Part print with two shaded views. Sizes in mm from the minimum x, y, z corner. A direction names the side the tool comes from. Coordinates: 2 decimals unless noted, no trailing zeros. Loops run counter-clockwise (first coordinate to the right, second up) from the corner with the lowest first, then second, coordinate; pieces in that order, holes last. Notation, with made-up numbers: (9.25, 19) -> (60.25, 19) arc R21 ccw to (60.25, 29) -> close; hole circle Ø5 at (-35, 54.5). An arc over 180 degrees is marked (long way). Answer as a JSON object with one key per item and string values. Group by question number.
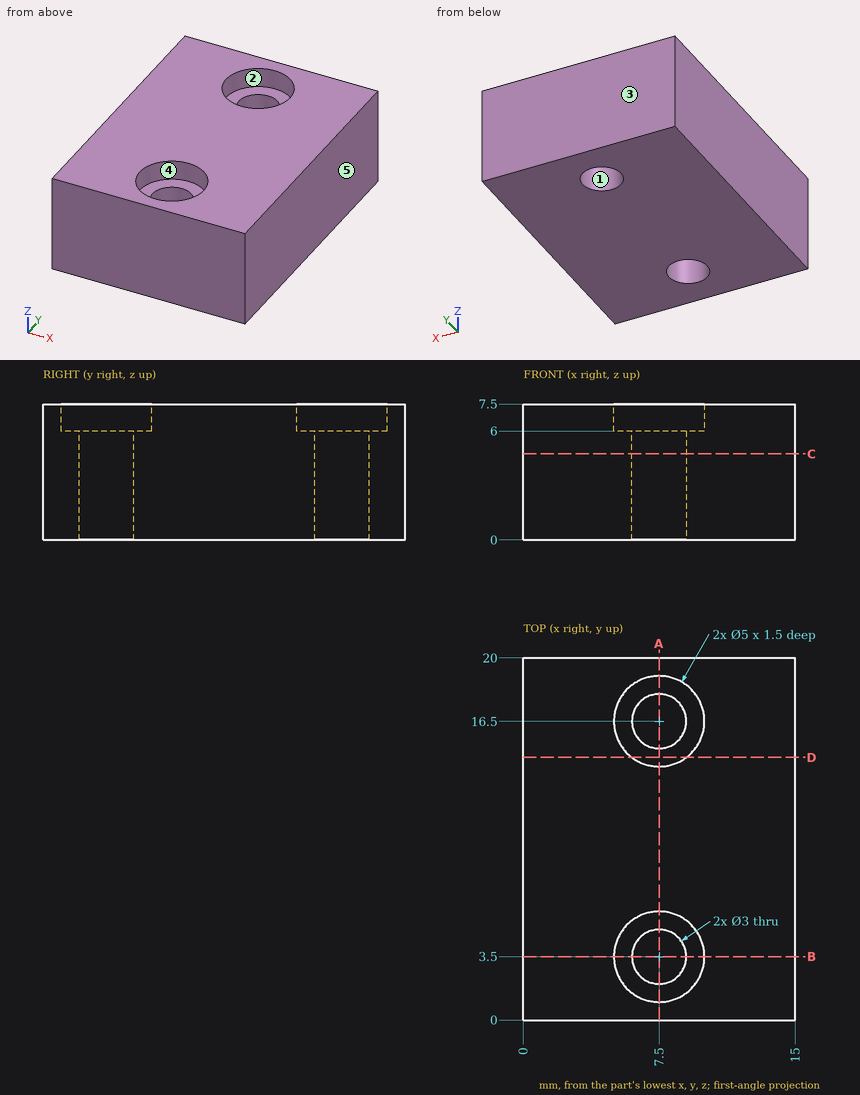
Item 1: Band-saw the part on D-D, the plane y = 14.5. List the corners of the cut face in (x, z).
Item 2: Band-saw the part on A-A, the plane x = 7.5. List the corners of the cut face in (y, z), and give its area (3 significant figures).
Item 3: Pull direction Y, two halves, no side cores. Call the marked faces 3, 4 and 5: +Y half, -Y half, draft (parallel to the pull), parting line (faces both ways), or undercut.
Item 4: 3-axis set-ups, long thin cutter, end or side, ignore diameter. For the marked faces 1 and 2: which of +Z, -Z, +X, -X, +Y, -Y reach the whole face in a straight line?
Item 5: Drill centre lines: L1, parallel to Y at x = 7.5, z = 3.4; L2, parallel to Y at x = 7.5, z = 6.4; L3, parallel to X at y = 4.5, z = 4.75. Where is each one in solid material? Low to high.
Item 6: Band-saw the part on C-C, the plane z = 4.75. List the corners of the cut face in (x, y).
Item 7: Band-saw the part on B-B, the plane y = 3.5. List the corners of the cut face in (x, z).
Item 8: Flat gauge pin, fed straight in: P1, Ø2.5, axis at x = 6.5, y = 16.5, coming from the +Z side. Where does the tip first touch, or does it go through?
Reply:
{
 "1": {"outline": "(0, 0) -> (15, 0) -> (15, 7.5) -> (9, 7.5) -> (9, 6) -> (6, 6) -> (6, 7.5) -> (0, 7.5) -> close"},
 "2": {"outline": "(0, 0) -> (2, 0) -> (2, 6) -> (1, 6) -> (1, 7.5) -> (0, 7.5) -> close; (5, 0) -> (15, 0) -> (15, 6) -> (14, 6) -> (14, 7.5) -> (6, 7.5) -> (6, 6) -> (5, 6) -> close; (18, 0) -> (20, 0) -> (20, 7.5) -> (19, 7.5) -> (19, 6) -> (18, 6) -> close", "area": "99.0 mm²"},
 "3": {"face 3": "+Y half", "face 4": "undercut", "face 5": "draft"},
 "4": {"face 1": "+Z, -Z", "face 2": "+Z"},
 "5": {"L1": "0 to 2, 5 to 15, 18 to 20", "L2": "0 to 1, 6 to 14, 19 to 20", "L3": "0 to 6.38, 8.62 to 15"},
 "6": {"outline": "(0, 0) -> (15, 0) -> (15, 20) -> (0, 20) -> close; hole circle Ø3 at (7.5, 3.5); hole circle Ø3 at (7.5, 16.5)"},
 "7": {"outline": "(0, 0) -> (6, 0) -> (6, 6) -> (5, 6) -> (5, 7.5) -> (0, 7.5) -> close; (9, 0) -> (15, 0) -> (15, 7.5) -> (10, 7.5) -> (10, 6) -> (9, 6) -> close"},
 "8": {"P1": "z = 6"}
}
